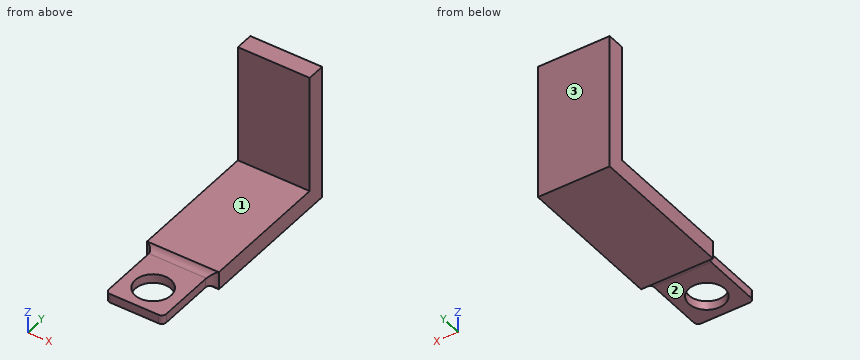
from build123d import *

# Parameters (mm, degrees)
SZKIC1_W                    = 4
SZKIC1_H                    = 1
DODANIE_WYCI_GNI_CIE1_DEPTH = 8.3
SZKIC2_W                    = 4
SZKIC2_H                    = 1
DODANIE_WYCI_GNI_CIE2_DEPTH = 6.6
SZKIC3_W                    = 3.2
SZKIC3_H                    = 0.5
DODANIE_WYCI_GNI_CIE3_DEPTH = 3.9
ZAOKR_GLENIE1_R             = 0.5
ZAOKR_GLENIE2_R             = 0.25
SZKIC4_R                    = 1
WYTNIJ_WYCI_GNI_CIE1_DEPTH  = 3.9


with BuildPart() as part:
    # Szkic1 → Dodanie-wyciągnięcie1 (new body)
    with BuildSketch(Plane(origin=(0, 0, 0), x_dir=(1, 0, 0), z_dir=(0, 1, 0))):
        with Locations((-2, -0.5)):
            Rectangle(SZKIC1_W, SZKIC1_H)
    extrude(amount=DODANIE_WYCI_GNI_CIE1_DEPTH)

    # Szkic2 → Dodanie-wyciągnięcie2 (add)
    with BuildSketch(Plane.XY.offset(1)):
        with Locations((-2, 7.8)):
            Rectangle(SZKIC2_W, SZKIC2_H)
    extrude(amount=DODANIE_WYCI_GNI_CIE2_DEPTH)

    # Szkic3 → Dodanie-wyciągnięcie3 (add)
    with BuildSketch(Plane.XZ):
        with Locations((-2, 0.5)):
            Rectangle(SZKIC3_W, SZKIC3_H)
    extrude(amount=DODANIE_WYCI_GNI_CIE3_DEPTH)

    # Zaokrąglenie1
    # the kernel refuses this fillet: 0.5 mm, written as the material it adds along each edge
    with BuildSketch(Plane(origin=(-0.4, 0, 0.25), x_dir=(1.0, -1.5702716904537035e-12, 0), z_dir=(0, 0, 1)), Plane(origin=(-3.6, 0, 0.75), x_dir=(-1.0, -1.5702716904537041e-12, 0), z_dir=(0, 0, -1))) as zaokr_glenie1_piece_1:
        with BuildLine():
            CenterArc((0.5, -0.489897949), ZAOKR_GLENIE1_R, 101.536959033, 78.463040967)
            Line((0, -0.489897949), (-0.01, -0.489897949))
            Line((-0.01, -0.489897949), (-0.01, 0))
            Line((-0.01, 0), (0, 0.01))
            ThreePointArc((0, 0.01), (0.2, 0.01), (0.398, 0.009797959))
            Line((0.398, 0.009797959), (0.4, 0))
        make_face()
    extrude(amount=0.5)
    with BuildSketch(Plane(origin=(-0.4, 0, 0.75), x_dir=(0, 0, 1), z_dir=(-1, 0, 0)), Plane(origin=(-3.6, 0, 0.25), x_dir=(0, 0, -1), z_dir=(1, 0, 0))) as zaokr_glenie1_piece_2:
        with BuildLine():
            CenterArc((0.5, -0.433012702), ZAOKR_GLENIE1_R, 120, 60)
            Line((0, -0.433012702), (-0.01, -0.433012702))
            Line((-0.01, -0.433012702), (-0.01, 0))
            Line((-0.01, 0), (0, 0.01))
            ThreePointArc((0, 0.01), (0.125, 0.01), (0.245, 0.008660254))
            Line((0.245, 0.008660254), (0.25, 0))
        make_face()
    extrude(amount=3.2)
    with BuildSketch(Plane(origin=(-0.4, 0, -0.974744871), x_dir=(1.0, -1.5702716904537035e-12, 0), z_dir=(0, 0, 1))) as zaokr_glenie1_piece_3a_section:
        with BuildLine():
            CenterArc((0.5, -0.489897949), ZAOKR_GLENIE1_R, 101.536959033, 78.463040967)
            Line((0, -0.489897949), (-0.01, -0.489897949))
            Line((-0.01, -0.489897949), (-0.01, 0))
            Line((-0.01, 0), (0, 0.01))
            ThreePointArc((0, 0.01), (0.2, 0.01), (0.398, 0.009797959))
            Line((0.398, 0.009797959), (0.4, 0))
        make_face()
    zaokr_glenie1_piece_3a = extrude(amount=1.724744871, mode=Mode.PRIVATE)
    zaokr_glenie1_piece_3a = split(zaokr_glenie1_piece_3a, bisect_by=Plane(origin=(-0.300219951, -0.114308546, 0), z_dir=(0, 0, 1)), keep=Keep.TOP, mode=Mode.PRIVATE)
    zaokr_glenie1_piece_3a = split(zaokr_glenie1_piece_3a, bisect_by=Plane(origin=(-0.300219951, -0.114308546, 0.25), z_dir=(0, 0, -1)), keep=Keep.TOP, mode=Mode.PRIVATE)
    with BuildSketch(Plane(origin=(-3.6, 0, 0.25), x_dir=(0, 0, -1), z_dir=(1, 0, 0))) as zaokr_glenie1_piece_3b_section:
        with BuildLine():
            CenterArc((0.5, -0.433012702), ZAOKR_GLENIE1_R, 120, 60)
            Line((0, -0.433012702), (-0.01, -0.433012702))
            Line((-0.01, -0.433012702), (-0.01, 0))
            Line((-0.01, 0), (0, 0.01))
            ThreePointArc((0, 0.01), (0.125, 0.01), (0.245, 0.008660254))
            Line((0.245, 0.008660254), (0.25, 0))
        make_face()
    zaokr_glenie1_piece_3b = extrude(amount=4.282531755, mode=Mode.PRIVATE)
    zaokr_glenie1_piece_3b = split(zaokr_glenie1_piece_3b, bisect_by=Plane(origin=(0, -0.108155223, 0.185241644), z_dir=(-1, 0, 0)), keep=Keep.TOP, mode=Mode.PRIVATE)
    zaokr_glenie1_piece_3b = split(zaokr_glenie1_piece_3b, bisect_by=Plane(origin=(-0.4, -0.108155223, 0.185241644), z_dir=(1, 0, 0)), keep=Keep.TOP, mode=Mode.PRIVATE)
    zaokr_glenie1_piece_3 = zaokr_glenie1_piece_3a & zaokr_glenie1_piece_3b
    add(zaokr_glenie1_piece_3)
    with BuildSketch(Plane(origin=(0.682531755, 0, 0.75), x_dir=(0, 0, 1), z_dir=(-1, 0, 0))) as zaokr_glenie1_piece_4a_section:
        with BuildLine():
            CenterArc((0.5, -0.433012702), ZAOKR_GLENIE1_R, 120, 60)
            Line((0, -0.433012702), (-0.01, -0.433012702))
            Line((-0.01, -0.433012702), (-0.01, 0))
            Line((-0.01, 0), (0, 0.01))
            ThreePointArc((0, 0.01), (0.125, 0.01), (0.245, 0.008660254))
            Line((0.245, 0.008660254), (0.25, 0))
        make_face()
    zaokr_glenie1_piece_4a = extrude(amount=4.282531755, mode=Mode.PRIVATE)
    zaokr_glenie1_piece_4a = split(zaokr_glenie1_piece_4a, bisect_by=Plane(origin=(0, -0.108155223, 0.814758356), z_dir=(-1, 0, 0)), keep=Keep.TOP, mode=Mode.PRIVATE)
    zaokr_glenie1_piece_4a = split(zaokr_glenie1_piece_4a, bisect_by=Plane(origin=(-0.4, -0.108155223, 0.814758356), z_dir=(1, 0, 0)), keep=Keep.TOP, mode=Mode.PRIVATE)
    with BuildSketch(Plane(origin=(-0.4, 0, 0.25), x_dir=(1.0, -1.5702716904537035e-12, 0), z_dir=(0, 0, 1))) as zaokr_glenie1_piece_4b_section:
        with BuildLine():
            CenterArc((0.5, -0.489897949), ZAOKR_GLENIE1_R, 101.536959033, 78.463040967)
            Line((0, -0.489897949), (-0.01, -0.489897949))
            Line((-0.01, -0.489897949), (-0.01, 0))
            Line((-0.01, 0), (0, 0.01))
            ThreePointArc((0, 0.01), (0.2, 0.01), (0.398, 0.009797959))
            Line((0.398, 0.009797959), (0.4, 0))
        make_face()
    zaokr_glenie1_piece_4b = extrude(amount=1.724744871, mode=Mode.PRIVATE)
    zaokr_glenie1_piece_4b = split(zaokr_glenie1_piece_4b, bisect_by=Plane(origin=(-0.300219951, -0.114308546, 1), z_dir=(0, 0, -1)), keep=Keep.TOP, mode=Mode.PRIVATE)
    zaokr_glenie1_piece_4b = split(zaokr_glenie1_piece_4b, bisect_by=Plane(origin=(-0.300219951, -0.114308546, 0.75), z_dir=(0, 0, 1)), keep=Keep.TOP, mode=Mode.PRIVATE)
    zaokr_glenie1_piece_4 = zaokr_glenie1_piece_4a & zaokr_glenie1_piece_4b
    add(zaokr_glenie1_piece_4)
    with BuildSketch(Plane(origin=(-3.6, 0, 1.974744871), x_dir=(-1.0, -1.5702716904537041e-12, 0), z_dir=(0, 0, -1))) as zaokr_glenie1_piece_5a_section:
        with BuildLine():
            CenterArc((0.5, -0.489897949), ZAOKR_GLENIE1_R, 101.536959033, 78.463040967)
            Line((0, -0.489897949), (-0.01, -0.489897949))
            Line((-0.01, -0.489897949), (-0.01, 0))
            Line((-0.01, 0), (0, 0.01))
            ThreePointArc((0, 0.01), (0.2, 0.01), (0.398, 0.009797959))
            Line((0.398, 0.009797959), (0.4, 0))
        make_face()
    zaokr_glenie1_piece_5a = extrude(amount=1.724744871, mode=Mode.PRIVATE)
    zaokr_glenie1_piece_5a = split(zaokr_glenie1_piece_5a, bisect_by=Plane(origin=(-3.699780049, -0.114308546, 1), z_dir=(0, 0, -1)), keep=Keep.TOP, mode=Mode.PRIVATE)
    zaokr_glenie1_piece_5a = split(zaokr_glenie1_piece_5a, bisect_by=Plane(origin=(-3.699780049, -0.114308546, 0.75), z_dir=(0, 0, 1)), keep=Keep.TOP, mode=Mode.PRIVATE)
    with BuildSketch(Plane(origin=(-0.4, 0, 0.75), x_dir=(0, 0, 1), z_dir=(-1, 0, 0))) as zaokr_glenie1_piece_5b_section:
        with BuildLine():
            CenterArc((0.5, -0.433012702), ZAOKR_GLENIE1_R, 120, 60)
            Line((0, -0.433012702), (-0.01, -0.433012702))
            Line((-0.01, -0.433012702), (-0.01, 0))
            Line((-0.01, 0), (0, 0.01))
            ThreePointArc((0, 0.01), (0.125, 0.01), (0.245, 0.008660254))
            Line((0.245, 0.008660254), (0.25, 0))
        make_face()
    zaokr_glenie1_piece_5b = extrude(amount=4.282531755, mode=Mode.PRIVATE)
    zaokr_glenie1_piece_5b = split(zaokr_glenie1_piece_5b, bisect_by=Plane(origin=(-4, -0.108155223, 0.814758356), z_dir=(1, 0, 0)), keep=Keep.TOP, mode=Mode.PRIVATE)
    zaokr_glenie1_piece_5b = split(zaokr_glenie1_piece_5b, bisect_by=Plane(origin=(-3.6, -0.108155223, 0.814758356), z_dir=(-1, 0, 0)), keep=Keep.TOP, mode=Mode.PRIVATE)
    zaokr_glenie1_piece_5 = zaokr_glenie1_piece_5a & zaokr_glenie1_piece_5b
    add(zaokr_glenie1_piece_5)
    with BuildSketch(Plane(origin=(-3.6, 0, 0.75), x_dir=(-1.0, -1.5702716904537041e-12, 0), z_dir=(0, 0, -1))) as zaokr_glenie1_piece_6a_section:
        with BuildLine():
            CenterArc((0.5, -0.489897949), ZAOKR_GLENIE1_R, 101.536959033, 78.463040967)
            Line((0, -0.489897949), (-0.01, -0.489897949))
            Line((-0.01, -0.489897949), (-0.01, 0))
            Line((-0.01, 0), (0, 0.01))
            ThreePointArc((0, 0.01), (0.2, 0.01), (0.398, 0.009797959))
            Line((0.398, 0.009797959), (0.4, 0))
        make_face()
    zaokr_glenie1_piece_6a = extrude(amount=1.724744871, mode=Mode.PRIVATE)
    zaokr_glenie1_piece_6a = split(zaokr_glenie1_piece_6a, bisect_by=Plane(origin=(-3.699780049, -0.114308546, 0), z_dir=(0, 0, 1)), keep=Keep.TOP, mode=Mode.PRIVATE)
    zaokr_glenie1_piece_6a = split(zaokr_glenie1_piece_6a, bisect_by=Plane(origin=(-3.699780049, -0.114308546, 0.25), z_dir=(0, 0, -1)), keep=Keep.TOP, mode=Mode.PRIVATE)
    with BuildSketch(Plane(origin=(-4.682531755, 0, 0.25), x_dir=(0, 0, -1), z_dir=(1, 0, 0))) as zaokr_glenie1_piece_6b_section:
        with BuildLine():
            CenterArc((0.5, -0.433012702), ZAOKR_GLENIE1_R, 120, 60)
            Line((0, -0.433012702), (-0.01, -0.433012702))
            Line((-0.01, -0.433012702), (-0.01, 0))
            Line((-0.01, 0), (0, 0.01))
            ThreePointArc((0, 0.01), (0.125, 0.01), (0.245, 0.008660254))
            Line((0.245, 0.008660254), (0.25, 0))
        make_face()
    zaokr_glenie1_piece_6b = extrude(amount=4.282531755, mode=Mode.PRIVATE)
    zaokr_glenie1_piece_6b = split(zaokr_glenie1_piece_6b, bisect_by=Plane(origin=(-4, -0.108155223, 0.185241644), z_dir=(1, 0, 0)), keep=Keep.TOP, mode=Mode.PRIVATE)
    zaokr_glenie1_piece_6b = split(zaokr_glenie1_piece_6b, bisect_by=Plane(origin=(-3.6, -0.108155223, 0.185241644), z_dir=(-1, 0, 0)), keep=Keep.TOP, mode=Mode.PRIVATE)
    zaokr_glenie1_piece_6 = zaokr_glenie1_piece_6a & zaokr_glenie1_piece_6b
    add(zaokr_glenie1_piece_6)

    # Zaokrąglenie2
    zaokr_glenie2_edges = [part.edges().sort_by_distance(p)[0] for p in [
        (-0.4, -3.9, 0.5),
        (-3.6, -3.9, 0.5),
    ]]
    fillet(zaokr_glenie2_edges, radius=ZAOKR_GLENIE2_R)

    # Szkic4 → Wytnij-wyciągnięcie1 (cut)
    with BuildSketch(Plane(origin=(0, 0, 0.25), x_dir=(-1, 0, 0), z_dir=(0, 0, -1))):
        with Locations((2, -2.399073148)):
            Circle(SZKIC4_R)
    extrude(amount=-WYTNIJ_WYCI_GNI_CIE1_DEPTH, mode=Mode.SUBTRACT)


solid = part.part
The listing builds one solid part. Answer for the finished solid, in the listing's coordinates (mm). Face numbers are marked on the shaded views. A direction names the side the tool comes from. Round coordinates to 2 decimals unless told otherwise and drop trailing zeros. Loops run counter-clockwise (first coordinate to the right, second up) from the corner with the lowest first, then second, coordinate; pieces in that order, holes last. Notation, with made-up numbers: M 17,-3 L 31,-3 A11 ccw 31,15 Z; hole C 9,55.5 d1. An arc over 180 degrees is marked long. Write each question's results on one line, items separated by ' | '. Start each with the question number.
1) Which of the six approach directions +Z, -Z, +X, -X, +Y, -Y give full straight-line access (tool end or side, diameter ignored) to the marked faces 1, 2 and 3?
2) Find section D-D on y = -0.75. Write down the section's boundary in (x, z), plus the area to 3 significant figures.
3) Straight lines are drawn through the part: probe 1 along Y at (x, z) = (-2, 0.45); probe 2 along Z at (x, y) = (-0.45, 4.75); probe 3 along Z at (x, y) = (-3, -1). For each, find the intervals that lie inside material, in ascending order.
4) Each of these flat-tipped pins is pushed along its axis until it touches: pin 1 (2 mm diameter, centred on x = -1.5, z = 6.5, fed in from -Y); pin 2 (0.6 mm diameter, centred on y = -2.5, z = 0.5, fed in from +X). Where does it stop, or does it pass through?
5) Find section B-B on x = -0.8. Write down the section's boundary in (y, z), plus the area to 3 significant figures.
6) Find section C-C on z = 6. Write down the section's boundary in (x, y).
7) Find section A-A on x = -2. Write down the section's boundary in (y, z).
Final values:
1) face 1: +Z, +X, -X, -Y | face 2: -Z, +X, -X, -Y | face 3: +Z, -Z, +X, -X, +Y
2) outline: M -3.6,0.25 L -0.4,0.25 L -0.4,0.75 L -3.6,0.75 Z | area: 1.60 mm²
3) probe 1: -3.9 to -3.4, -1.4 to 8.3 | probe 2: 0 to 1 | probe 3: 0.25 to 0.75
4) pin 1: y = 7.3 | pin 2: x = -0.4
5) outline: M -3.9,0.25 L -0.43,0.25 A0.5 cw 0,0 L 8.3,0 L 8.3,7.6 L 7.3,7.6 L 7.3,1 L 0,1 A0.5 cw -0.43,0.75 L -3.9,0.75 Z | area: 16.9 mm²
6) outline: M -4,7.3 L 0,7.3 L 0,8.3 L -4,8.3 Z
7) outline: M -3.9,0.25 L -3.4,0.25 L -3.4,0.75 L -3.9,0.75 Z; M -1.4,0.25 L -0.43,0.25 A0.5 cw 0,0 L 8.3,0 L 8.3,7.6 L 7.3,7.6 L 7.3,1 L 0,1 A0.5 cw -0.43,0.75 L -1.4,0.75 Z
